```python
from build123d import *

# Parameters (mm, degrees)
F0_W     = 150
F0_H     = 10
F1_DEPTH = 90
F2_T     = -2.5
F3_R     = 12.538546
F4_DEPTH = 25


with BuildPart() as f1:
    # F0 (on Top) → F1 (new body)
    with BuildSketch(Plane.XY):
        Rectangle(F0_W, F0_H)
    extrude(amount=F1_DEPTH)

    # F2
    f2_openings = [f1.faces().sort_by_distance(p)[0] for p in [
        (0, 0, 0),
    ]]
    offset(amount=F2_T, openings=f2_openings)

    # F3 (on face) → F4 (cut)
    with BuildSketch(Plane.XZ.offset(5)):
        with Locations((0, 90)):
            Circle(F3_R)
    extrude(amount=-F4_DEPTH, mode=Mode.SUBTRACT)


solid = f1.part
```
Can you work these out from the model? Positions are in its coordinate system, mm. A direction names the side the tool comes from. Coordinates: 2 decimals unless noted, no trailing zeros. Loops run counter-clockwise (first coordinate to the right, second up) from the corner with the lowest first, then second, coordinate; pieces in that order, holes last.
1) For pin 1 (2.5 mm diameter, centred on x = -43.5, y = -1, fed in from -Z); pin 2 (5.5 mm diameter, centred on x = 52.5, y = 0, fed in from -Z), each with a flat end and sliding along its axis, tell me the tip position at first contact or that it passes through.
2) Imagine slicing it at C-C on z = 40. List the corners of the cut face in (x, y) for me, plus the area to 3 significant figures.
3) Imagine slicing it at A-A on y = 1. List the corners of the cut face in (x, z) for me, plus the area to 3 significant figures.
4) Imagine slicing it at D-D on x = 15. List the corners of the cut face in (y, z) for me.
5) I need wall thicknesses on probe 1 along X at (y, z) = (1.5, 20.5); probe 2 along Y at (x, z) = (51.5, 42); probe 3 along Z at (x, y) = (45.5, -0.25). Which ranges of each line are inside material? Lowest first, please.
6) Thinking about a two-plate mould opening in X: for faces 1 (the flat face through (-75, 0, 44)), 2 (the flat face through (-43, 0, 87.5)), 3 (the flat face through (43, 0, 90)), which applies, pulls with the +X half, pulls with the -X half, needs draft (parallel to the pull), parting line crosses it, or undercut?
7) Imagine slicing it at B-B on x = 0. List the corners of the cut face in (y, z) for me, plus the area to 3 significant figures.
8) Which directions (+Z, -Z, +X, -X, +Y, -Y) give clear straight access to the entire face, cutting with the end or side of a thin tool? Please do faces 4 (the flat face through (-1, 2.5, 43)), 5 (the flat face through (-1, 5, 44)).
Completed:
1. pin 1: stops at z = 87.5
1. pin 2: stops at z = 0
2. outline: (-75, -5) - (75, -5) - (75, 5) - (-75, 5) - close; hole (-72.5, -2.5) - (72.5, -2.5) - (72.5, 2.5) - (-72.5, 2.5) - close
2. area: 775 mm2
3. outline: (-75, 0) - (-72.5, 0) - (-72.5, 87.5) - (-12.29, 87.5) arc R12.54 cw to (-12.54, 90) - (-75, 90) - close; (12.29, 87.5) - (72.5, 87.5) - (72.5, 0) - (75, 0) - (75, 90) - (12.54, 90) arc R12.54 cw to start
3. area: 750 mm2
4. outline: (-5, 0) - (-2.5, 0) - (-2.5, 87.5) - (2.5, 87.5) - (2.5, 0) - (5, 0) - (5, 90) - (-5, 90) - close
5. probe 1: x = -75 to -72.5, 72.5 to 75
5. probe 2: y = -5 to -2.5, 2.5 to 5
5. probe 3: z = 87.5 to 90
6. face 1: pulls with the -X half
6. face 2: undercut
6. face 3: needs draft
7. outline: (-5, 0) - (-2.5, 0) - (-2.5, 77.46) - (-5, 77.46) - close; (2.5, 0) - (5, 0) - (5, 77.46) - (2.5, 77.46) - close
7. area: 387 mm2
8. face 4: -Z
8. face 5: +Z, -Z, +X, -X, +Y
